from build123d import *

# Parameters (mm, degrees)
F1_DEPTH = 6
F3_DEPTH = 4
F5_DEPTH = 5
F6_W     = 13
F6_H     = 3.4
F7_DEPTH = 10
F9_DEPTH = 14.4


# Not quite as in the source:
# - a feature names something its author has since deleted; it is built from what else it names


with BuildPart() as f1:
    # F0 (on Top) → F1 (new body)
    with BuildSketch(Plane.XY):
        with BuildLine():
            ThreePointArc((0, 3.3761399509), (0.1464466094, 3.0225865603), (0.5, 2.8761399509))
            Line((0.5, 2.8761399509), (13.9, 2.8761399509))
            ThreePointArc((13.9, 2.8761399509), (14.2535533906, 3.0225865603), (14.4, 3.3761399509))
            Line((14.4, 3.3761399509), (0, 3.3761399509))
        make_face()
        with BuildLine():
            Line((0, 12.3761399509), (0, 3.3761399509))
            Line((0, 3.3761399509), (14.4, 3.3761399509))
            Line((14.4, 3.3761399509), (14.4, 12.3761399509))
            ThreePointArc((14.4, 12.3761399509), (13.9606601718, 13.4368001227), (12.9, 13.8761399509))
            Line((12.9, 13.8761399509), (1.5, 13.8761399509))
            ThreePointArc((1.5, 13.8761399509), (0.4393398282, 13.4368001227), (0, 12.3761399509))
        make_face()
        with BuildLine():
            ThreePointArc((3, 11.3761399509), (3.2928932188, 12.0832467321), (4, 12.3761399509))
            Line((4, 12.3761399509), (10.4, 12.3761399509))
            ThreePointArc((10.4, 12.3761399509), (11.1071067812, 12.0832467321), (11.4, 11.3761399509))
            Line((11.4, 11.3761399509), (11.4, 10.5761399509))
            ThreePointArc((11.4, 10.5761399509), (11.1071067812, 9.8690331698), (10.4, 9.5761399509))
            Line((10.4, 9.5761399509), (4, 9.5761399509))
            ThreePointArc((4, 9.5761399509), (3.2928932188, 9.8690331698), (3, 10.5761399509))
            Line((3, 10.5761399509), (3, 11.3761399509))
        make_face(mode=Mode.SUBTRACT)
    extrude(amount=F1_DEPTH)

    # F2 (on Top) → F3 (cut)
    with BuildSketch(Plane.XY):
        with BuildLine():
            ThreePointArc((13.9, 11.8761399509), (13.4606601718, 12.9368001227), (12.4, 13.3761399509))
            Line((12.4, 13.3761399509), (2, 13.3761399509))
            ThreePointArc((2, 13.3761399509), (0.9393398282, 12.9368001227), (0.5, 11.8761399509))
            Line((0.5, 11.8761399509), (0.5, 4.8761399509))
            ThreePointArc((0.5, 4.8761399509), (0.9393398282, 3.8154797792), (2, 3.3761399509))
            Line((2, 3.3761399509), (12.4, 3.3761399509))
            ThreePointArc((12.4, 3.3761399509), (13.4606601718, 3.8154797792), (13.9, 4.8761399509))
            Line((13.9, 4.8761399509), (13.9, 11.8761399509))
        make_face()
    extrude(amount=F3_DEPTH, mode=Mode.SUBTRACT)

    # F4 (on face) → F5 (join)
    with BuildSketch(Plane.XY.offset(6)):
        with BuildLine():
            Line((14.4, 6.6761399509), (0, 6.6761399509))
            Line((0, 6.6761399509), (0, 3.3761399509))
            ThreePointArc((0, 3.3761399509), (0.1464466094, 3.0225865603), (0.5, 2.8761399509))
            Line((0.5, 2.8761399509), (13.9, 2.8761399509))
            ThreePointArc((13.9, 2.8761399509), (14.2535533906, 3.0225865603), (14.4, 3.3761399509))
            Line((14.4, 3.3761399509), (14.4, 6.6761399509))
        make_face()
    extrude(amount=F5_DEPTH)

    # F6 (on face) → F7 (cut)
    with BuildSketch(Plane(origin=(0, 0, 0), x_dir=(1, 0, 0), z_dir=(0, 0, -1))):
        with Locations((7.2, -4.7761399509)):
            Rectangle(F6_W, F6_H)
    extrude(amount=-F7_DEPTH, mode=Mode.SUBTRACT)

    # F8 (on Right) → F9 (join)
    with BuildSketch(Plane.YZ):
        with BuildLine():
            add(Edge.make_bspline(
                [(7.1272827151, 6), (6.8833303011, 6.9959140901), (6.6957208529, 9.2354907336), (6.6761399509, 11)],
                knots=[0.4613630388, 0.4613630388, 0.4613630388, 0.4613630388, 1, 1, 1, 1], degree=3))
            Line((6.6761399509, 11), (6.6761399509, 6))
            Line((6.6761399509, 6), (7.1272827151, 6))
        make_face()
        with BuildLine():
            add(Edge.make_bspline(
                [(7.9261399509, 6), (7.8912804031, 6.0110682928), (7.8586101723, 6.0100642713), (7.8278293535, 6)],
                knots=[0, 0, 0, 0, 0.0376755281, 0.0376755281, 0.0376755281, 0.0376755281], degree=3))
            Line((7.8278293535, 6), (7.9261399509, 6))
        make_face()
        with BuildLine():
            Line((7.8278293535, 6), (7.1272827151, 6))
            add(Edge.make_bspline(
                [(7.8278293535, 6), (7.6417958125, 5.9391734168), (7.4240615582, 5.2101966849), (7.2160450595, 5.6376356026), (7.1272827151, 6)],
                knots=[0.0376755281, 0.0376755281, 0.0376755281, 0.0376755281, 0.2653794095, 0.4613630388, 0.4613630388, 0.4613630388, 0.4613630388], degree=3))
        make_face()
    extrude(amount=F9_DEPTH)


solid = f1.part
Geometry check sheet. Reference: the model listing, model coordinates, mm. A direction names the side the tool comes from. Give positions to 0.01 mm unless a question says otherwise; leave off trailing zeros. Write each loop counter-clockwise with the first axis right and the second up, starting at its lowest first coordinate (ties: lowest second). Pieces come first, ordered by that corner, then holes. Notation, with made-up numbers: M -10,-5 L 3,-5 A29 ccw 3,26 Z; hole C -35.5,-30.5 d6. An arc over 180 degrees is marked long. One line per question, with ' | ' between items.
1. Set-up check for faces 1 (the face through (0, 7, 4)), 2 (the face through (13.9, 8, 2)), 3 (the face through (7, 9.576, 5)): record each of +Z, -Z, +X, -X, +Y, -Y from which the full face is reachable in a straight line by a thin tool's end or side.
Ans:
face 1: +Z, -Z, -X, +Y, -Y | face 2: -Z | face 3: +Z, -Z
2. Cross-section at C-C (z = 5.75). Enter the section's corners in (x, y).
Ans:
outline: M 0,3.38 A0.5 ccw 0.5,2.88 L 13.9,2.88 A0.5 ccw 14.4,3.38 L 14.4,12.38 A1.5 ccw 12.9,13.88 L 1.5,13.88 A1.5 ccw 0,12.38 Z; hole M 0.7,3.08 L 13.7,3.08 L 13.7,6.48 L 0.7,6.48 Z; hole M 3,10.58 A1 ccw 4,9.58 L 10.4,9.58 A1 ccw 11.4,10.58 L 11.4,11.38 A1 ccw 10.4,12.38 L 4,12.38 A1 ccw 3,11.38 Z
3. Cross-section at D-D (y = 6). Enter the section's corners in (x, z), plus the area to 3 significant figures.
Ans:
outline: M 0,0 L 0.5,0 L 0.5,4 L 0.7,4 L 0.7,10 L 13.7,10 L 13.7,4 L 13.9,4 L 13.9,0 L 14.4,0 L 14.4,11 L 0,11 Z | area: 26.8 mm2
4. Mould release check, pull along Y, two halves, no side actions. Record for faces 4 (the face through (7, 2.876, 5)), 5 (the face through (7, 13, 6)), 6 (the face through (11.1, 12.09, 4.99)), 7 (the face through (11.4, 11, 5)): released by +Y, released by -Y, zero draft, split by the parting line, or undercut.
Ans:
face 4: released by -Y | face 5: zero draft | face 6: undercut | face 7: undercut
5. Cross-section at A-A (z = 1). Enter the section's corners in (x, y).
Ans:
outline: M 0,3.38 A0.5 ccw 0.5,2.88 L 13.9,2.88 A0.5 ccw 14.4,3.38 L 14.4,12.38 A1.5 ccw 12.9,13.88 L 1.5,13.88 A1.5 ccw 0,12.38 Z; hole M 0.5,4.88 A1.5 ccw 0.7,4.13 L 0.7,3.08 L 13.7,3.08 L 13.7,4.13 A1.5 ccw 13.9,4.88 L 13.9,11.88 A1.5 ccw 12.4,13.38 L 2,13.38 A1.5 ccw 0.5,11.88 Z
6. Scan lines: line 1 along Y through (x, z) = (6.75, 5.5); line 2 along Y through (x, z) = (6.25, 0.75); line 3 along Y through (x, z) = (3.75, 4.25). Record each from-to range of solid material in increasing order. Write a range as from..to.
Ans:
line 1: 2.88..3.08, 6.48..9.58, 12.38..13.88 | line 2: 2.88..3.08, 13.38..13.88 | line 3: 2.88..3.08, 6.48..9.61, 12.34..13.88
7. Cross-section at B-B (y = 9.25). Enter the section's corners in (x, z).
Ans:
outline: M 0,0 L 0.5,0 L 0.5,4 L 13.9,4 L 13.9,0 L 14.4,0 L 14.4,6 L 0,6 Z
8. Gauge pin test, flat ends, axial feed: pin 1 (1.8 mm diameter, centred on x = 4.5, y = 11, fed in from +Z); pin 2 (1 mm diameter, centred on x = 13, y = 5.5, fed in from -Z); pin 3 (1 mm diameter, centred on x = 11.5, y = 11, fed in from +Z). Record the tip position at first contact, or that the pin passes through.
Ans:
pin 1: through | pin 2: z = 10 | pin 3: z = 6
